The model under review builds one solid part; all positions refer to its coordinate system, in mm. Face numbers are marked on the shaded views. A direction names the side the tool comes from. Round coordinates to 2 decimals unless told otherwise and drop trailing zeros. Write each loop counter-clockwise with the first axis right and the second up, starting at its lowest first coordinate (ties: lowest second). Pieces come first, ordered by that corner, then holes. Notation, with made-up numbers: (46.5, -26) - (99.5, -26) arc R33 cw to (99.5, 13) - close; hole circle Ø4 at (85, 4). An arc over 180 degrees is marked (long way). Use one line per item in the form item = value.
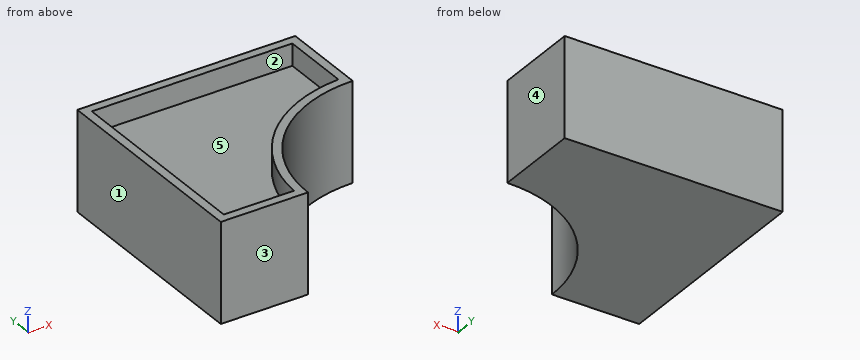
from build123d import *

# Parameters (mm, degrees)
BOSS_EXTRUDE2_DEPTH = 28.956
CUT_EXTRUDE1_DEPTH  = 6.35


with BuildPart() as part:
    # Sketch1 → Boss-Extrude2 (new body)
    with BuildSketch(Plane.XY):
        with BuildLine():
            Line((0, 0), (63.5, 0))
            Line((63.5, 0), (63.5, -25.4))
            ThreePointArc((63.5, -25.4), (36.559231637, -36.559231637), (25.4, -63.5))
            Line((25.4, -63.5), (0, -63.5))
            Line((0, -63.5), (0, 0))
        make_face()
    extrude(amount=BOSS_EXTRUDE2_DEPTH)

    # Sketch2 → Cut-Extrude1 (cut)
    with BuildSketch(Plane.XY.offset(28.956)):
        with BuildLine():
            Line((2.54, -2.54), (2.54, -60.96))
            Line((2.54, -60.96), (22.939452666, -60.96))
            ThreePointArc((22.939452666, -60.96), (34.763180413, -34.763180413), (60.96, -22.939452666))
            Line((60.96, -22.939452666), (60.96, -2.54))
            Line((60.96, -2.54), (2.54, -2.54))
        make_face()
    extrude(amount=-CUT_EXTRUDE1_DEPTH, mode=Mode.SUBTRACT)


solid = part.part
(1) Add section C-C on y = -14.5. Write out the cut boundary in (x, z), then the cut area to 3 significant figures.
Geometry results:
outline = (0, 0) - (63.5, 0) - (63.5, 28.96) - (60.96, 28.96) - (60.96, 22.61) - (2.54, 22.61) - (2.54, 28.96) - (0, 28.96) - close
area = 1,470 mm2
(2) Add section B-B on x = 14. Write out the cut boundary in (y, z).
Geometry results:
outline = (-63.5, 0) - (0, 0) - (0, 28.96) - (-2.54, 28.96) - (-2.54, 22.61) - (-60.96, 22.61) - (-60.96, 28.96) - (-63.5, 28.96) - close
(3) Machinability: for the marked faces 1 and 2, which of the approach directions +Z, -Z, +X, -X, +Y, -Y give a long, thin tool a straight path to every point of the face, cutting with its end or side? Answer none if there is none.
Geometry results:
face_1 = +Z, -Z, -X, +Y, -Y
face_2 = +Z
(4) Add section D-D on z = 17.5. Write out the cut boundary in (x, y).
Geometry results:
outline = (0, -63.5) - (25.4, -63.5) arc R38.1 cw to (63.5, -25.4) - (63.5, 0) - (0, 0) - close
(5) To check wall thickness, follow L1, parallel to Y at x = 15.5, z = 27; L2, parallel to Z at x = 33, y = -28.5; L3, parallel to Y at x = 41, z = 25.75. State the ranges of each line that lie inside material, in increasing order.
Geometry results:
L1 = -63.5 to -60.96, -2.54 to 0
L2 = 0 to 22.61
L3 = -32.75 to -29.66, -2.54 to 0
(6) The part is to be moulded in two halves that separate along Y. For the marked faces 3, 4 and 5, say which applies: +Y half, -Y half, draft (parallel to the pull), parting line (faces both ways), or undercut.
Geometry results:
face_3 = -Y half
face_4 = draft
face_5 = undercut
(7) Insertion check: P1, Ø1.9, axis at y = -38, z = 27, coming from the +X side; P2, Ø5, axis at x = 18, y = -55, coming from the +Z side. Each pin has a flat end and moves straight along its axis. Give the tip position at first contact, or say it passes through.
Geometry results:
P1 = 36.08
P2 = 22.61
(8) Add section A-A on z = 26.5. Write out the cut boundary in (x, y), then the cut area to 3 significant figures.
Geometry results:
outline = (0, -63.5) - (25.4, -63.5) arc R38.1 cw to (63.5, -25.4) - (63.5, 0) - (0, 0) - close; hole (2.54, -60.96) - (22.94, -60.96) arc R40.64 cw to (60.96, -22.94) - (60.96, -2.54) - (2.54, -2.54) - close
area = 577 mm2
